```python
from build123d import *

# Parameters (mm, degrees)
ESQUISSE1_W             = 40
ESQUISSE1_H             = 7
BOSS_EXTRU_1_DEPTH      = 5
ENL_V_MAT_EXTRU_2_DEPTH = 6
ESQUISSE4_W             = 40
ESQUISSE4_H             = 3
BOSS_EXTRU_2_DEPTH      = 6
ESQUISSE5_R             = 1.625
ENL_V_MAT_EXTRU_3_DEPTH = 6
ESQUISSE6_W             = 15
ESQUISSE6_H             = 3
BOSS_EXTRU_3_DEPTH      = 50
ESQUISSE7_W             = 10
ESQUISSE7_H             = 3
BOSS_EXTRU_4_DEPTH      = 13.2
ESQUISSE8_W             = 30
ESQUISSE8_H             = 10
BOSS_EXTRU_5_DEPTH      = 20
ESQUISSE9_W             = 29.4
ESQUISSE9_H             = 18.4
ESQUISSE9_W_2           = 23.4
ESQUISSE9_H_2           = 12.4
BOSS_EXTRU_6_DEPTH      = 15
ESQUISSE11_W            = 10
ESQUISSE11_H            = 5
ENL_V_MAT_EXTRU_5_DEPTH = 15


with BuildPart() as part:
    # Esquisse1 → Boss.-Extru.1 (new body)
    with BuildSketch(Plane.XY):
        with Locations((20, -3.5)):
            Rectangle(ESQUISSE1_W, ESQUISSE1_H)
    extrude(amount=BOSS_EXTRU_1_DEPTH)

    # Esquisse3 → Enlèv. mat.-Extru.2 (cut, through all)
    with BuildSketch(Plane.XY.offset(5)):
        Polygon((40, 0), (0, 0), (0, -1.5), align=None)
    extrude(amount=-ENL_V_MAT_EXTRU_2_DEPTH, mode=Mode.SUBTRACT)

    # Esquisse4 → Boss.-Extru.2 (add)
    with BuildSketch(Plane(origin=(0, 0, 0), x_dir=(-1, 0, 0), z_dir=(0, 0, -1))):
        with Locations((-20, -5.5)):
            Rectangle(ESQUISSE4_W, ESQUISSE4_H)
    extrude(amount=BOSS_EXTRU_2_DEPTH)

    # Esquisse5 → Enlèv. mat.-Extru.3 (cut)
    with BuildSketch(Plane(origin=(0, -4, 0), x_dir=(1, 0, 0), z_dir=(0, 1, 0))):
        with Locations((35, 2.949699752)):
            Circle(ESQUISSE5_R)
        with Locations((5, 2.949699752)):
            Circle(ESQUISSE5_R)
    extrude(amount=-ENL_V_MAT_EXTRU_3_DEPTH, mode=Mode.SUBTRACT)

    # Esquisse6 → Boss.-Extru.3 (add)
    with BuildSketch(Plane(origin=(0, 0, -6), x_dir=(-1, 0, 0), z_dir=(0, 0, -1))):
        with Locations((-7.5, -5.5)):
            Rectangle(ESQUISSE6_W, ESQUISSE6_H)
    extrude(amount=BOSS_EXTRU_3_DEPTH)

    # Esquisse7 → Boss.-Extru.4 (add)
    with BuildSketch(Plane.ZY):
        with Locations((-51, -5.5)):
            Rectangle(ESQUISSE7_W, ESQUISSE7_H)
    extrude(amount=BOSS_EXTRU_4_DEPTH)

    # Esquisse8 → Boss.-Extru.5 (add)
    with BuildSketch(Plane(origin=(0, -4, 0), x_dir=(1, 0, 0), z_dir=(0, 1, 0))):
        with Locations((1.8, 51)):
            Rectangle(ESQUISSE8_W, ESQUISSE8_H)
    extrude(amount=BOSS_EXTRU_5_DEPTH)

    # Esquisse9 → Boss.-Extru.6 (add)
    with BuildSketch(Plane.XY.offset(-46)):
        with Locations((1.5, 5.2)):
            Rectangle(ESQUISSE9_W, ESQUISSE9_H)
        with Locations((1.5, 5.2)):
            Rectangle(ESQUISSE9_W_2, ESQUISSE9_H_2, mode=Mode.SUBTRACT)
    extrude(amount=BOSS_EXTRU_6_DEPTH)

    # Esquisse11 → Enlèv. mat.-Extru.5 (cut)
    with BuildSketch(Plane(origin=(0, 0, -56), x_dir=(-1, 0, 0), z_dir=(0, 0, -1))):
        with Locations((8.2, 5.5)):
            Rectangle(ESQUISSE11_W, ESQUISSE11_H)
    extrude(amount=-ENL_V_MAT_EXTRU_5_DEPTH, mode=Mode.SUBTRACT)


solid = part.part
```
The listing builds one solid part. Answer for the finished solid, in the listing's coordinates (mm). A direction names the side the tool comes from. Give positions to 0.01 mm unless a question says otherwise; leave off trailing zeros. Order: outer loops, then holes, each group sorted by start corner. A loop starts at its lowest first (then second) coordinate and runs counter-clockwise, first axis right, second up. Notation, with made-up numbers: (66.5, 76.25) -> (91.5, 76.25) arc R28 ccw to (91.5, 107.25) -> close; hole circle Ø10 at (1.25, 55.5). An arc over 180 degrees is marked (long way). Write each question's results on one line, items separated by ' | '.
Q1. The part is cut by section C-C, the plane x = -2. Give the vertices of the cut face in (y, z), and give its area (3 significant figures).
Checked values:
outline: (-7, -56) -> (16, -56) -> (16, -46) -> (14.4, -46) -> (14.4, -31) -> (11.4, -31) -> (11.4, -46) -> (-1, -46) -> (-1, -31) -> (-4, -31) -> (-4, -46) -> (-7, -46) -> close | area: 320 mm^2
Q2. The part is cut by section A-A, the plane z = -39. Give the vertices of the cut face in (x, y).
Checked values:
outline: (-13.2, -4) -> (0, -4) -> (0, -7) -> (15, -7) -> (15, -4) -> (16.2, -4) -> (16.2, 14.4) -> (-13.2, 14.4) -> close; hole (-10.2, -1) -> (13.2, -1) -> (13.2, 11.4) -> (-10.2, 11.4) -> close
Q3. Straight lines are drawn through the part: probe 1 along X at (y, z) = (4.25, -38.5); probe 2 along Y at (x, z) = (-7.5, -38); probe 3 along Z at (x, y) = (35, -5.65). For each, find the intervals that lie inside material, in ascending order. Write a range as from..to.
Checked values:
probe 1: x = -13.2..-10.2, 13.2..16.2 | probe 2: y = -4..-1, 11.4..14.4 | probe 3: z = -6..-4.57, -1.32..5
Q4. The part is cut by section B-B, the plane x = 35. Give the vertices of the cut face in (y, z).
Checked values:
outline: (-7, -6) -> (-4, -6) -> (-4, -4.57) -> (-7, -4.57) -> close; (-7, -1.32) -> (-4, -1.32) -> (-4, 0) -> (-0.19, 0) -> (-0.19, 5) -> (-7, 5) -> close
Q5. Determine the mould class of faces 1 (the face through (-10.2, 5, -37)), 2 (the face through (16.8, 6, -51)), 3 (the face through (1, 14.4, -39)) for opening direction X: pulls with the +X half, pulls with the -X half, needs draft (parallel to the pull), parting line crosses it, or undercut.
Checked values:
face 1: undercut | face 2: pulls with the +X half | face 3: needs draft
Q6. Each of these flat-tipped pins is pushed along its axis until it touches: P1, Ø7.5, axis at x = -3, z = -35, coming from the +Y side; P2, Ø10, axis at y = 5.5, z = -37, coming from the +X side; P3, Ø1, axis at x = 13.5, y = 9.5, coming from the +Z side. Where does it stop, or does it pass through?
Checked values:
P1: stops at y = 14.4 | P2: stops at x = 16.2 | P3: stops at z = -31
Q7. Which of the six approach directions +Z, -Z, +X, -X, +Y, -Y give full straight-line access (tool end or side, diameter ignored) to faces 4 (the face through (-8, 8, -50)), 5 (the face through (15, -6, -31)), 6 (the face through (1, -1, -39)), 7 (the face through (19.72, -0.76, 2.54))?
Checked values:
face 4: -Z, -X | face 5: -Z, +X, -Y | face 6: +Z | face 7: +Z, -X, +Y
Q8. The part is cut by section D-D, the plane y = 1.5. Give the vertices of the cut face in (x, z), and give its area (3 significant figures).
Checked values:
outline: (-13.2, -56) -> (16.8, -56) -> (16.8, -46) -> (16.2, -46) -> (16.2, -31) -> (13.2, -31) -> (13.2, -46) -> (-10.2, -46) -> (-10.2, -31) -> (-13.2, -31) -> close | area: 390 mm^2
